```python
from build123d import *

# Parameters (mm, degrees)
F1_DEPTH = 57.6
F2_DEPTH = 5
F3_START = -5
F3_DEPTH = 5


# Not quite as in the source:
# - a feature names something its author has since deleted; it is built from what else it names


with BuildPart() as f1:
    # F0 (on Right) → F1 (new body)
    with BuildSketch(Plane.YZ):
        Polygon((1.5365748771, 3.633035603), (0, 0), (20.4984284937, 0), (11.0311029763, 26.0816380962), align=None)
        Polygon((0, 4.2829225325), (0, 0), (1.5365748771, 3.633035603), align=None)
        Polygon((-1.811441418, 0), (0, 0), (0, 4.2829225325), align=None)
        Polygon((-1.811441418, 0), (0, 4.2829225325), (-1.1518723498, 4.7701013845), (-3.1693637124, 0), align=None)
    extrude(amount=F1_DEPTH)

    # F0 (on Right) → F2 (join)
    with BuildSketch(Plane.YZ):
        Polygon((-1.1518723498, 4.7701013845), (0, 4.2829225325), (9.4668246651, 26.666023784), (10.1944775948, 28.3864664644), (9.5673128152, 30.1142495409), (8.3149523153, 27.153202636), align=None)
        Polygon((1.5365748771, 3.633035603), (0, 0), (20.4984284937, 0), (11.0311029763, 26.0816380962), align=None)
        Polygon((-1.811441418, 0), (0, 0), (0, 4.2829225325), align=None)
        Polygon((-1.811441418, 0), (0, 4.2829225325), (-1.1518723498, 4.7701013845), (-3.1693637124, 0), align=None)
        Polygon((0, 4.2829225325), (0, 0), (1.5365748771, 3.633035603), align=None)
    extrude(amount=-F2_DEPTH)

    # F0 (on Right) → F3 (join)
    with BuildSketch(Plane.YZ.offset(F3_START)):
        Polygon((-1.1518723498, 4.7701013845), (0, 4.2829225325), (9.4668246651, 26.666023784), (10.1944775948, 28.3864664644), (9.5673128152, 30.1142495409), (8.3149523153, 27.153202636), align=None)
        Polygon((0, 4.2829225325), (1.5365748771, 3.633035603), (11.0311029763, 26.0816380962), (10.1944775948, 28.3864664644), (9.4668246651, 26.666023784), align=None)
        Polygon((1.5365748771, 3.633035603), (0, 0), (20.4984284937, 0), (11.0311029763, 26.0816380962), align=None)
        Polygon((0, 4.2829225325), (0, 0), (1.5365748771, 3.633035603), align=None)
        Polygon((-1.811441418, 0), (0, 0), (0, 4.2829225325), align=None)
        Polygon((-1.811441418, 0), (0, 4.2829225325), (-1.1518723498, 4.7701013845), (-3.1693637124, 0), align=None)
    extrude(amount=-F3_DEPTH)


solid = f1.part
```
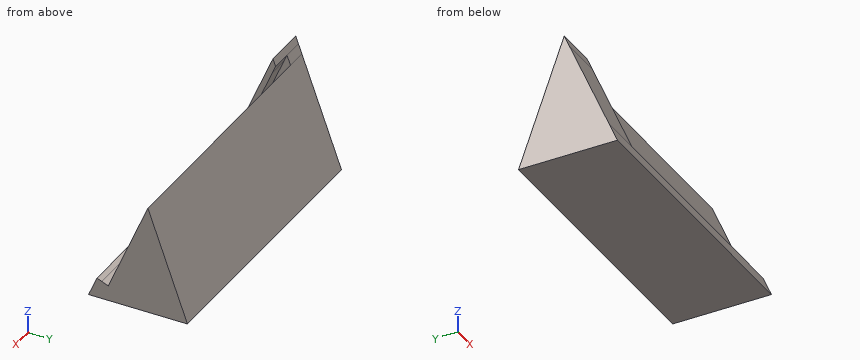
Can you work these out from the model? Positions are in its coordinate system, mm. Coordinates: 2 decimals unless noted, no trailing zeros. Loops run counter-clockwise (first coordinate to the right, second up) from the corner with the lowest first, then second, coordinate; pieces in that order, holes last. Notation, with made-up numbers: (36, 7) - (88, 7) arc R16 ccw to (88, 29) - close; hole circle Ø7 at (-22, 85.5). An arc over 180 degrees is marked (long way). Use a Markdown table: item, result.
Item 1: I want a section at C-C on y = 4.25. Please give me the cut outline in (x, z).
Numbers:
| item | result |
|---|---|
| outline | (-10, 0) - (57.6, 0) - (57.6, 10.05) - (-5, 10.05) - (-5, 14.33) - (0, 14.33) - (0, 17.54) - (-10, 17.54) - close |
Item 2: I want a section at B-B on z = 12.5. Please give me the cut outline in (x, y), and give its area (3 significant figures).
Numbers:
| item | result |
|---|---|
| outline | (-10, 2.12) - (0, 2.12) - (0, 3.48) - (-5, 3.48) - (-5, 5.29) - (57.6, 5.29) - (57.6, 15.96) - (-10, 15.96) - close |
| area | 744 mm2 |
Item 3: I want a section at A-A on x = -1. Please give me the cut outline in (y, z).
Numbers:
| item | result |
|---|---|
| outline | (-3.17, 0) - (20.5, 0) - (11.03, 26.08) - (1.54, 3.63) - (0, 4.28) - (10.19, 28.39) - (9.57, 30.11) - close |
Item 4: I want a section at D-D on x = 7. Please give me the cut outline in (y, z), and give its area (3 significant figures).
Numbers:
| item | result |
|---|---|
| outline | (-3.17, 0) - (20.5, 0) - (11.03, 26.08) - (1.54, 3.63) - (-1.15, 4.77) - close |
| area | 281 mm2 |
Item 5: If I drill on probe 1 along X at (y, z) = (1, 9); probe 2 along Y at (x, z) = (33, 4); probe 3 along Z at (x, y) = (-1.5, 7.5), over which ranges is the centre line in solid material (lowest first)? Write a range as from..to.
Numbers:
| item | result |
|---|---|
| probe 1 | x = -10..0 |
| probe 2 | y = -1.48..0.67, 1.69..19.05 |
| probe 3 | z = 0..17.73, 22.02..25.23 |
Item 6: Will these pins go through, and if not, where does the flat tip stop? pin 1 (4 mm diameter, centred on x = 47, z = 19, fed in from +Y); pin 2 (8 mm diameter, centred on x = 36.5, z = 23.5, fed in from +Y); pin 3 (1.5 mm diameter, centred on x = 48.5, z = 22, fed in from -Y).
Numbers:
| item | result |
|---|---|
| pin 1 | stops at y = 14.33 |
| pin 2 | stops at y = 13.42 |
| pin 3 | stops at y = 8.99 |
